from build123d import *

# Parameters (mm, degrees)
SKETCH_W = 1
SKETCH_H = 5


with BuildPart() as part:
    # AdditivePipe: sweep along a path in Sketch001
    with BuildLine(Plane.XY) as additivepipe_path:
        Line((0, 0), (10, 0))
        ThreePointArc((10, 0), (11.62655, 0.60151), (12.470399, 2.116567))
        Line((12.470399, 2.116567), (14.529557, 15.383433))
        ThreePointArc((14.529557, 15.383433), (17.109663, 17.497593), (19.494501, 15.16539))
        Line((19.494501, 15.16539), (21.505454, -15.165388))
        ThreePointArc((21.505454, -15.165388), (23.999977, -17.5), (26.494501, -15.165389))
        Line((26.494501, -15.165389), (28.505454, 15.165389))
        ThreePointArc((28.505454, 15.165389), (30.999978, 17.5), (33.494501, 15.165388))
        Line((33.494501, 15.165388), (35.505455, -15.16539))
        ThreePointArc((35.505455, -15.16539), (37.890292, -17.497593), (40.470399, -15.383433))
        Line((40.470399, -15.383433), (42.529557, -2.116567))
        ThreePointArc((42.529557, -2.116567), (43.373406, -0.60151), (44.999956, 0))
        Line((44.999956, 0), (54.999956, 0))
    # Sketch → AdditivePipe (sweep)
    with BuildSketch(Plane.YZ):
        with Locations((0, 2.5)):
            Rectangle(SKETCH_W, SKETCH_H)
    sweep(path=additivepipe_path.line)


solid = part.part
Could you check a few things on this model? Use its own coordinates, in mm. A direction names the side the tool comes from. Give positions to 0.01 mm unless a question says otherwise; leave off trailing zeros. Write each loop counter-clockwise with the first axis right and the second up, starting at its lowest first coordinate (ties: lowest second). Pieces come first, ordered by that corner, then holes. Notation, with made-up numbers: (-14, 82) - (11, 82) arc R38 cw to (11, 120) - close; hole circle Ø4 at (32, 81). An arc over 180 degrees is marked (long way). Use CSV: the item, a comma, the result in double quotes. Start each with the question number.
Item 1: I want a section at A-A, the plane y = -7.5. Please give me the cut outline in (x, z).
Item 2: I want a section at B-B, the plane z = 3.15. Please give me the cut outline in (x, y), then the cut area to 3 significant figures.
Item 3: If I drill on line 1 along X through (y, z) = (-9, 2.7); line 2 along X through (y, z) = (-1.5, 1.55); line 3 along Y through (x, z) = (45, 0.5), over which ranges is the centre line in solid material (lowest first)?
Item 4: I want a section at C-C, the plane x = 39. Please give me the cut outline in (y, z).
Item 5: I'm going to push flat-ended pins straight in: pin 1 (8 mm diameter, centred on x = 13, y = 13.5, fed in from -Z); pin 2 (1.5 mm diameter, centred on x = 50.5, z = 2.5, fed in from -Y); pin 3 (2 mm diameter, centred on x = 14.5, z = 0.5, fed in from +Y); pin 4 (2.5 mm diameter, centred on x = 48.5, z = 1.5, fed in from +Y). Where does each tip first touch, or does it pass through?
Item 6: For faces 4 (the face through (21, 0, 2)), 5 (the face through (50, 0.5, 2)), 6 (the face through (20, 0, 3)), 7 (the face through (50, -0.5, 3)), 8 (the face through (5, -0.5, 3)), which set-ups out of +Z, -Z, +X, -X, +Y, -Y let a thin tool reach every point of the face, with its end or its side?
Item 7: If we mould it in two halves opening along X, with no side actions, what happens to faces 1 (the face through (35, 0, 2)), 2 (the face through (13.02, 8.92, 2.47)), 3 (the face through (42.01, -8.73, 2.54))? For each: pulls with the +X half, pulls with the -X half, needs draft (parallel to the pull), parting line crosses it, or undercut.
Findings:
1,outline,"(20.5, 0) - (21.5, 0) - (21.5, 5) - (20.5, 5) - close; (26.5, 0) - (27.5, 0) - (27.5, 5) - (26.5, 5) - close; (34.5, 0) - (35.5, 0) - (35.5, 5) - (34.5, 5) - close; (41.19, 0) - (42.2, 0) - (42.2, 5) - (41.19, 5) - close"
2,outline,"(0, -0.5) - (10, -0.5) arc R3 ccw to (12.96, 2.04) - (15.02, 15.31) arc R2 cw to (19, 15.13) - (21.01, -15.2) arc R3 ccw to (26.99, -15.2) - (29, 15.13) arc R2 cw to (33, 15.13) - (35.01, -15.2) arc R3 ccw to (40.96, -15.46) - (43.02, -2.19) arc R2 cw to (45, -0.5) - (55, -0.5) - (55, 0.5) - (45, 0.5) arc R3 ccw to (42.04, -2.04) - (39.98, -15.31) arc R2 cw to (36, -15.13) - (33.99, 15.2) arc R3 ccw to (28.01, 15.2) - (26, -15.13) arc R2 cw to (22, -15.13) - (19.99, 15.2) arc R3 ccw to (14.04, 15.46) - (11.98, 2.19) arc R2 cw to (10, 0.5) - (0, 0.5) - close"
2,area,"175 mm2"
3,line 1,"x = 20.6 to 21.6, 26.4 to 27.4, 34.6 to 35.6, 40.96 to 41.97"
3,line 2,"x = 20.1 to 21.1, 26.9 to 27.9, 34.1 to 35.1, 42.17 to 43.27"
3,line 3,"y = -0.5 to 0.5"
4,outline,"(-17.83, 0) - (-16.73, 0) - (-16.73, 5) - (-17.83, 5) - close"
5,pin 1,"stops at z = 0"
5,pin 2,"stops at y = -0.5"
5,pin 3,"stops at y = 17.6"
5,pin 4,"stops at y = 0.5"
6,face 4,"+Z, -Z, +Y"
6,face 5,"+Z, -Z, +X, +Y"
6,face 6,"+Z, -Z, -Y"
6,face 7,"+Z, -Z, +X, -Y"
6,face 8,"+Z, -Z, -X, -Y"
7,face 1,"undercut"
7,face 2,"pulls with the -X half"
7,face 3,"pulls with the +X half"
